```python
from build123d import *

# Parameters (mm, degrees)
F0_W     = 51
F0_H     = 40
F1_DEPTH = 41
F4_W     = 5.5
F4_H     = 40
F5_DEPTH = 30
F7_DEPTH = 30
F2_R     = 2.5
F8_DEPTH = 41.001
F9_D     = 8.4
F9_DEPTH = 20
F9_TIP   = 2.5236145999


with BuildPart() as f1:
    # F0 (on Front) → F1 (new body)
    with BuildSketch(Plane.XZ):
        Rectangle(F0_W, F0_H)
    extrude(amount=F1_DEPTH)

    # F4 (on face) → F5 (cut)
    with BuildSketch(Plane.XZ.offset(41)):
        with Locations((22.75, 0)):
            Rectangle(F4_W, F4_H)
        with Locations((-22.75, 0)):
            Rectangle(F4_W, F4_H)
    extrude(amount=-F5_DEPTH, mode=Mode.SUBTRACT)

    # F6 (on face) → F7 (cut)
    with BuildSketch(Plane.XZ.offset(41)):
        with BuildLine():
            Line((-20, 20), (-20, 17.1716884745))
            ThreePointArc((-20, 17.1716884745), (-23.5355339059, 8.6361545685), (-15, 12.1716884745))
            Line((-15, 12.1716884745), (-15, 20))
            Line((-15, 20), (-20, 20))
        make_face()
        with BuildLine():
            Line((20, 17.1716884745), (20, 20))
            Line((20, 20), (15, 20))
            Line((15, 20), (15, 12.1716884745))
            ThreePointArc((15, 12.1716884745), (23.5355339059, 8.6361545685), (20, 17.1716884745))
        make_face()
        with BuildLine():
            Line((20, -20), (20, -17.1716884745))
            ThreePointArc((20, -17.1716884745), (23.5355339059, -8.6361545685), (15, -12.1716884745))
            Line((15, -12.1716884745), (15, -20))
            Line((15, -20), (20, -20))
        make_face()
        with BuildLine():
            ThreePointArc((-15, -12.1716884745), (-23.5355339059, -8.6361545685), (-20, -17.1716884745))
            Line((-20, -17.1716884745), (-20, -20))
            Line((-20, -20), (-15, -20))
            Line((-15, -20), (-15, -12.1716884745))
        make_face()
    extrude(amount=-F7_DEPTH, mode=Mode.SUBTRACT)

    # F2 (on face) → F8 (cut, through all)
    with BuildSketch(Plane(origin=(0, 0, 0), x_dir=(-1, 0, 0), z_dir=(0, 1, 0))):
        with Locations((-20, 12)):
            Circle(F2_R)
        with Locations((-20, -12)):
            Circle(F2_R)
        with Locations((20, -12)):
            Circle(F2_R)
        with Locations((20, 12)):
            Circle(F2_R)
    extrude(amount=-F8_DEPTH, mode=Mode.SUBTRACT)

    # F9
    with Locations(Plane.XZ.offset(41)):
        with Locations((-14, 0), (14, 0)):
            Hole(F9_D / 2, depth=F9_DEPTH)
            with Locations((0, 0, -(F9_DEPTH + F9_TIP / 2))):  # 118° drill point
                Cone(0, F9_D / 2, F9_TIP, mode=Mode.SUBTRACT)


solid = f1.part
```
Verification items for the finished model (mm, model axes). A direction names the side the tool comes from. Coordinates: 2 decimals unless noted, no trailing zeros. Loops run counter-clockwise (first coordinate to the right, second up) from the corner with the lowest first, then second, coordinate; pieces in that order, holes last. Notation, with made-up numbers: (50, 82.25) -> (96, 82.25) arc R25 ccw to (96, 103.25) -> close; hole circle Ø10 at (-4, 85). An arc over 180 degrees is marked (long way). Put each result on its own line as item: value.
1. Mould release check, pull along X, two halves, no side actions. Record for faces 1 (the face through (25.5, -5, 0)), 2 (the face through (-16.4, -26.2, -8.7)), 3 (the face through (18.196, -30.86, 0.185)): pulls with the +X half, pulls with the -X half, needs draft (parallel to the pull), parting line crosses it, or undercut.
Result set:
face 1: pulls with the +X half
face 2: pulls with the -X half
face 3: undercut
2. Tool access check on faces 4 (the face through (-16.5, -26.2, 8.6)), 5 (the face through (16.5, -26.2, -8.6)), 6 (the face through (-15, -26, -16)). Record the directions out of +Z, -Z, +X, -X, +Y, -Y that give a thin tool (end or side, any length) a straight path to the whole face; none if there is none.
Result set:
face 4: +Z, -X, -Y
face 5: -Z, +X, -Y
face 6: -Z, -X, -Y
3. Section check A-A, the plane y = -35. Record the boundary of the cut face in (x, z).
Result set:
outline: (-20, -7.17) arc R5 cw to (-15, -12.17) -> (-15, -20) -> (15, -20) -> (15, -12.17) arc R5 cw to (20, -7.17) -> (20, 7.17) arc R5 cw to (15, 12.17) -> (15, 20) -> (-15, 20) -> (-15, 12.17) arc R5 cw to (-20, 7.17) -> close; hole circle Ø8.4 at (-14, 0); hole circle Ø8.4 at (14, 0)
4. Section check C-C, the plane y = -17.5. Record the boundary of the cut face in (x, z), then the cut area to 3 significant figures.
Result set:
outline: (-20, -7.17) arc R5 cw to (-15, -12.17) -> (-15, -20) -> (15, -20) -> (15, -12.17) arc R5 cw to (20, -7.17) -> (20, 7.17) arc R5 cw to (15, 12.17) -> (15, 20) -> (-15, 20) -> (-15, 12.17) arc R5 cw to (-20, 7.17) -> close
area: 1,360 mm^2
5. Thickness scan on line 1 (Z direction, x = 20, y = -8.75); line 2 (X direction, y = -30, z = 0); line 3 (Z direction, x = 14, y = -29.5). Record the ranges inside material, lowest first.
Result set:
line 1: z = -20 to -14.5, -9.5 to 9.5, 14.5 to 20
line 2: x = -20 to -18.2, -9.8 to 9.8, 18.2 to 20
line 3: z = -20 to -4.2, 4.2 to 20
6. Gauge pin test, flat ends, axial feed: P1, Ø5, axis at x = -14, z = 0, coming from the -Y side; P2, Ø4, axis at y = -23, z = -16, coming from the -X side; P3, Ø1.5, axis at y = -24, z = -2.5, coming from the +X side; P4, Ø3, axis at x = -20, z = 12, coming from the +Y side. Record the tip position at first contact, or that the pin passes through.
Result set:
P1: stops at y = -19.98
P2: stops at x = -15
P3: stops at x = 20
P4: passes through
7. Section check B-B, the plane x = -19. Record the boundary of the cut face in (y, z).
Result set:
outline: (-41, -7.27) -> (-11, -7.27) -> (-11, -9.71) -> (0, -9.71) -> (0, 9.71) -> (-11, 9.71) -> (-11, 7.27) -> (-41, 7.27) -> close; (-11, -20) -> (0, -20) -> (0, -14.29) -> (-11, -14.29) -> close; (-11, 14.29) -> (0, 14.29) -> (0, 20) -> (-11, 20) -> close
